The model under review builds one solid part; all positions refer to its coordinate system, in mm. A direction names the side the tool comes from. Coordinates: 2 decimals unless noted, no trailing zeros. Write each loop counter-clockwise with the first axis right and the second up, starting at its lowest first coordinate (ties: lowest second). Pieces come first, ordered by that corner, then holes. Notation, with made-up numbers: M -7,0 L -3,0 A28 ccw -3,32 Z; hole C 69,19.25 d9. An arc over 180 degrees is marked long. Answer as a JSON object with one key per item and string values.
```python
from build123d import *

# Parameters (mm, degrees)
SKETCH1_W           = 20
SKETCH1_H           = 88
SKETCH1_R           = 1.5
BOSS_EXTRUDE1_DEPTH = 5
SKETCH2_W           = 20
SKETCH2_H           = 5
BOSS_EXTRUDE2_DEPTH = 144
FILLET1_R           = 8
SKETCH3_R           = 1.939400698
CUT_EXTRUDE1_DEPTH  = 6


with BuildPart() as part:
    # Sketch1 → Boss-Extrude1 (new body)
    with BuildSketch(Plane.XY):
        with Locations((10, 44)):
            Rectangle(SKETCH1_W, SKETCH1_H)
        with Locations((14, 82)):
            Circle(SKETCH1_R, mode=Mode.SUBTRACT)
        with Locations((14, 23)):
            Circle(SKETCH1_R, mode=Mode.SUBTRACT)
    extrude(amount=BOSS_EXTRUDE1_DEPTH)

    # Sketch2 → Boss-Extrude2 (add)
    with BuildSketch(Plane.XY.offset(5)):
        with Locations((10, 2.5)):
            Rectangle(SKETCH2_W, SKETCH2_H)
    extrude(amount=BOSS_EXTRUDE2_DEPTH)

    # Fillet1
    fillet1_edges = [part.edges().sort_by_distance(p)[0] for p in [
        (20, 88, 2.5),
        (0, 88, 2.5),
    ]]
    fillet(fillet1_edges, radius=FILLET1_R)

    # Sketch3 → Cut-Extrude1 (cut, through all)
    with BuildSketch(Plane(origin=(0, 5, 0), x_dir=(1, 0, 0), z_dir=(0, 1, 0))):
        with Locations((14, -143)):
            Circle(SKETCH3_R)
        with Locations((14, -11)):
            Circle(SKETCH3_R)
    extrude(amount=-CUT_EXTRUDE1_DEPTH, mode=Mode.SUBTRACT)


solid = part.part
```
(1) Add section D-D on z = 102.5. Give the boundary of the cut face in (x, y).
Results list:
{"outline": "M 0,0 L 20,0 L 20,5 L 0,5 Z"}
(2) Add section B-B on x = 14. Give the boundary of the cut face in (y, z).
Results list:
{"outline": "M 0,0 L 21.5,0 L 21.5,5 L 5,5 L 5,9.06 L 0,9.06 Z; M 0,12.94 L 5,12.94 L 5,141.06 L 0,141.06 Z; M 0,144.94 L 5,144.94 L 5,149 L 0,149 Z; M 24.5,0 L 80.5,0 L 80.5,5 L 24.5,5 Z; M 83.5,0 L 87.75,0 L 87.75,5 L 83.5,5 Z"}
(3) For pin 1 Ø5 at (x, z) = (14, 37.5) entering from -Y; pin 2 Ø6 at (x, z) = (11.5, 111.5) entering from +Y; pin 3 Ø8 at (x, y) = (17, 28) entering from +Z, all flat-tipped, find the tip position at first contact; note any pin that passes through.
Results list:
{"pin 1": "y = 0", "pin 2": "y = 5", "pin 3": "z = 5"}
(4) Wall thickness on line 1 along Z through (x, y) = (14, 2.05); line 2 along X through (y, z) = (3.65, 143); line 3 along Y through (x, z) = (14, 1.85): over which ranges is each line inside the solid? List them lowest first. Write a range as from..to.
Results list:
{"line 1": "0..9.06, 12.94..141.06, 144.94..149", "line 2": "0..12.06, 15.94..20", "line 3": "0..21.5, 24.5..80.5, 83.5..87.75"}
(5) Add section A-A on z = 11. Give the boundary of the cut face in (x, y).
Results list:
{"outline": "M 0,0 L 12.06,0 L 12.06,5 L 0,5 Z; M 15.94,0 L 20,0 L 20,5 L 15.94,5 Z"}
(6) For faces 5 (the face through (2.281, 85.594, 2.535)), 6 (the face through (10, 5, 76)), list the 3-axis set-ups (+Z, -Z, +X, -X, +Y, -Y) from which the entire face can be reached by the end or side of a thin tool; tool diameter is ignored.
Results list:
{"face 5": "+Z, -Z, -X, +Y", "face 6": "+Z, +X, -X, +Y"}
(7) Add section C-C on y = 23. Give the boundary of the cut face in (x, z).
Results list:
{"outline": "M 0,0 L 12.5,0 L 12.5,5 L 0,5 Z; M 15.5,0 L 20,0 L 20,5 L 15.5,5 Z"}
(8) Draft analysis for pull direction X (two halves, no side actions). For faces 1 (the face through (13.58, 2.535, 144.893)), 2 (the face through (15.043, 2.535, 9.365)), 3 (the face through (17.719, 85.594, 2.535)), 4 (the face through (10, 47, 5)), state which applies: released by +X, released by -X, zero draft, split by the parting line, or undercut.
Results list:
{"face 1": "undercut", "face 2": "undercut", "face 3": "released by +X", "face 4": "zero draft"}
